```python
from build123d import *

# Parameters (mm, degrees)
F0_W      = 420
F0_H      = 290
F1_DEPTH  = 12
F2_W      = 12
F2_H      = 290
F3_DEPTH  = 880
F7_W      = 420
F7_H      = 290
F8_DEPTH  = 12
F9_W      = 420
F9_H      = 290
F10_DEPTH = 12
F13_W     = 420
F13_H     = 290
F14_DEPTH = 12
F15_W     = 420
F15_H     = 892
F16_DEPTH = 12


with BuildPart() as f1:
    # F0 (on Top) → F1 (new body)
    with BuildSketch(Plane.XY):
        with Locations((210, 145)):
            Rectangle(F0_W, F0_H)
    extrude(amount=F1_DEPTH)

    # F2 (on face) → F3 (join)
    with BuildSketch(Plane.XY.offset(12)):
        with Locations((6, 145)):
            Rectangle(F2_W, F2_H)
        with Locations((414, 145)):
            Rectangle(F2_W, F2_H)
    extrude(amount=F3_DEPTH)

    # F7 (on offset) → F8 (join)
    with BuildSketch(Plane.XY.offset(300)):
        with Locations((210, 145)):
            Rectangle(F7_W, F7_H)
    extrude(amount=F8_DEPTH)

    # F9 (on offset) → F10 (join)
    with BuildSketch(Plane.XY.offset(600)):
        with Locations((210, 145)):
            Rectangle(F9_W, F9_H)
    extrude(amount=F10_DEPTH)

    # F13 (on 3pt) → F14 (join)
    with BuildSketch(Plane(origin=(0, 0, 892), x_dir=(1, 0, 0), z_dir=(0, 0, -1))):
        with Locations((210, -145)):
            Rectangle(F13_W, F13_H)
    extrude(amount=F14_DEPTH)

    # F15 (on face) → F16 (join)
    with BuildSketch(Plane(origin=(0, 290, 0), x_dir=(-1, 0, 0), z_dir=(0, 1, 0))):
        with Locations((-210, 446)):
            Rectangle(F15_W, F15_H)
    extrude(amount=F16_DEPTH)


solid = f1.part
```
Build history of the part. All positions in model axes, mm. A direction names the side the tool comes from. Round coordinates to 2 decimals unless told otherwise and drop trailing zeros. Write each loop counter-clockwise with the first axis right and the second up, starting at its lowest first coordinate (ties: lowest second). Pieces come first, ordered by that corner, then holes.
1) Band-saw the part on C-C, the plane z = 199. List the corners of the cut face in (x, y).
2) Drill centre lines: probe 1 along Z at (x, y) = (138, 71); probe 2 along X at (y, z) = (103, 664); probe 3 along Y at (x, z) = (237.5, 198). Where is each one in solid material? Low to high.
3) Mould opens along X. For faces 1 (the flat face through (12, 143, 744)), 2 (the flat face through (408, 143, 154)), 3 (the flat face through (213, 302, 452)), 4 (the flat face through (420, 149, 440)) say: +X half, -X half, draft (parallel to the pull), parting line (faces both ways), or undercut.
4) Band-saw the part on B-B, the plane x = 343. List the corners of the cut face in (y, z).
5) 3-axis set-ups, long thin cutter, end or side, ignore diameter. For faces 5 (the flat face through (213, 149, 0)), 6 (the flat face through (207, 147, 600)): which of +Z, -Z, +X, -X, +Y, -Y reach the whole face in a straight line?
6) Band-saw the part on A-A, the plane y = 80. List the corners of the cut face in (x, z).
Ans:
1. outline: (0, 0) - (12, 0) - (12, 290) - (408, 290) - (408, 0) - (420, 0) - (420, 302) - (0, 302) - close
2. probe 1: z = 0 to 12, 300 to 312, 600 to 612, 880 to 892
2. probe 2: x = 0 to 12, 408 to 420
2. probe 3: y = 290 to 302
3. face 1: undercut
3. face 2: undercut
3. face 3: draft
3. face 4: +X half
4. outline: (0, 0) - (302, 0) - (302, 892) - (0, 892) - (0, 880) - (290, 880) - (290, 612) - (0, 612) - (0, 600) - (290, 600) - (290, 312) - (0, 312) - (0, 300) - (290, 300) - (290, 12) - (0, 12) - close
5. face 5: -Z, +X, -X, +Y, -Y
5. face 6: -Y
6. outline: (0, 0) - (420, 0) - (420, 892) - (0, 892) - close; hole (12, 12) - (408, 12) - (408, 300) - (12, 300) - close; hole (12, 312) - (408, 312) - (408, 600) - (12, 600) - close; hole (12, 612) - (408, 612) - (408, 880) - (12, 880) - close
